Work out the finished part from the listing and answer in its coordinate system (mm). Face numbers are marked on the shaded views. A direction names the side the tool comes from. Round coordinates to 2 decimals unless told otherwise and drop trailing zeros. Write each loop counter-clockwise with the first axis right and the second up, starting at its lowest first coordinate (ties: lowest second). Pieces come first, ordered by that corner, then holes. Notation, with made-up numbers: (29, 16) -> (46, 16) arc R19 cw to (46, 39) -> close; hole circle Ø1 at (-36.5, 63). An arc over 180 degrees is marked (long way). One line per item, written item: value.
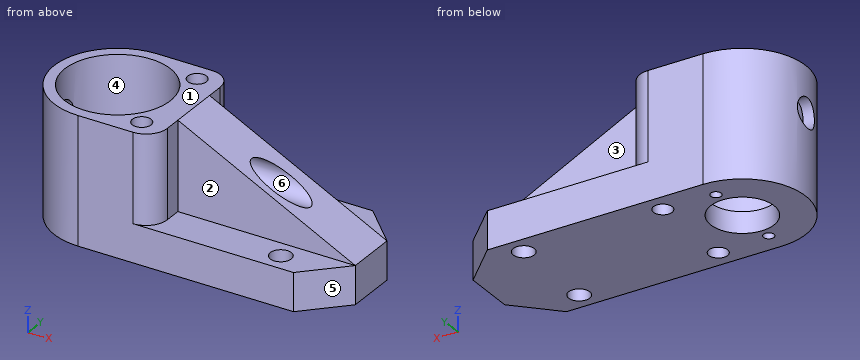
Autodesk Fusion 360 part; units mm, degrees
sketch "Sketch1" plane through (0, 0, 0) normal (0, 1, 0) x (1, 0, 0)
sketch "Sketch2" plane through (0, 0, 0) normal (0, 0, 1) x (1, 0, 0)
  line L0 (30, 15) -> (-30, 15)
  line L1 (-30, 15) -> (-30, -15)
  line L2 (-30, -15) -> (30, -15)
  line L3 (30, -15) -> (30, 15)
  line L4 (30, 15) -> (-30, -15) construction
  line L5 (-30, 15) -> (30, -15) construction
  arc A0 (-30, 15) -> (-30, -15) centre (-30, 0) ccw
  circle A1 centre (-30, 0) radius 7.5
  line L6 (21, -15) -> (30, -6)
  line L7 (21, 15) -> (30, 6)
  dimension "d1" = 60
  dimension "d2" = 30
  dimension "d3" = 15
  dimension "d4" = 9
  dimension "d5" = 9
  dimension "d6" = 9
  dimension "d7" = 9
extrude "Extrude1" add sketch "Sketch2" along normal blind 9 contours L0 L1 L2 L3 A1 L6 L7 | L1 A0 A1
sketch "Sketch3" plane through (0, 0, 9) normal (0, 0, 1) x (-1, 0, 0)
  circle A0 centre (30, 0) radius 7.5
  arc A1 (30, -15) -> (30, 15) centre (30, 0) ccw
  line L0 (30, 15) -> (-21, 15)
  line L1 (-21, 15) -> (-30, 6)
  line L2 (-30, 6) -> (-30, -6)
  line L3 (-30, -6) -> (-21, -15)
  line L4 (-21, -15) -> (30, -15)
  line L5 (12, 15) -> (12, -15)
  dimension "d10" = 18
extrude "Extrude2" add sketch "Sketch3" along normal blind 21 contours A1 L0 L4 L5
sketch "Sketch4" plane through (0, 0, 0) normal (0, 1, 0) x (1, 0, 0)
  line L0 (30, -9) -> (-12, -30)
  line L1 (-12, -30) -> (-12, -9)
  line L2 (-12, -9) -> (30, -9)
extrude "Extrude3" add sketch "Sketch4" along normal mid plane 12
sketch "Sketch5" plane through (0, 0, 30) normal (0, 0, 1) x (-1, 0, 0)
  circle A0 centre (30, 0) radius 7.5
  line L0 (12, 15) -> (12, 6)
  line L1 (12, 6) -> (12, -6)
  line L2 (12, -6) -> (12, -15)
  line L3 (12, -15) -> (30, -15)
  arc A1 (30, -15) -> (30, 15) centre (30, 0) ccw
  line L4 (30, 15) -> (12, 15)
  circle A2 centre (17.7307, -10.5) radius 2.2228
  circle A3 centre (17.7307, -10.5) radius 2.5
  dimension "d15" = 5
extrude "Extrude4" cut sketch "Sketch5" against normal blind 30 contours A2
mirror "Mirror1" about plane through (0, 0, 0) normal (0, 1, 0) of "Extrude4"
sketch "Sketch6" plane through (0, 0, 30) normal (0, 0, 1) x (-1, 0, 0)
  circle A0 centre (17.7307, 10.5) radius 2.2228
  circle A1 centre (17.7307, -10.5) radius 2.2228
  circle A2 centre (30, 0) radius 7.5
  line L0 (12, 15) -> (12, 6)
  line L1 (12, 6) -> (12, -6)
  line L2 (12, -6) -> (12, -15)
  line L3 (12, -15) -> (30, -15)
  arc A3 (30, -15) -> (30, 15) centre (30, 0) ccw
  line L4 (30, 15) -> (12, 15)
  circle A4 centre (30, 0) radius 12.5
  dimension "d20" = 25
extrude "Extrude5" cut sketch "Sketch6" against normal blind 25 contours A4
sketch "Sketch7" plane through (0, 0, 5) normal (0, 0, 1) x (-1, 0, 0)
  circle A0 centre (30, 0) radius 7.5
  circle A1 centre (30, 0) radius 12.5
  circle A2 centre (30, 10) radius 1.25
  dimension "d23" = 2.5
extrude "Extrude6" cut sketch "Sketch7" against normal blind 5 contours A2
sketch "Sketch8" plane through (0, 0, 5) normal (0, 0, 1) x (-1, 0, 0)
  circle A0 centre (30, 10) radius 1.25
  circle A1 centre (30, 0) radius 7.5
  circle A2 centre (30, 0) radius 12.5
  circle A3 centre (30, -10) radius 1.25
  dimension "d26" = 2.5
extrude "Extrude7" cut sketch "Sketch8" against normal blind 5 contours A3
sketch "Sketch9" plane through (0, 0, 0) normal (0, 0, -1) x (1, 0, 0)
  circle A0 centre (-30, -10) radius 1.25
  circle A1 centre (-30, 10) radius 1.25
  circle A2 centre (-17.7307, 10.5) radius 2.2228
  circle A3 centre (-17.7307, -10.5) radius 2.2228
  circle A4 centre (-30, 0) radius 7.5
  arc A5 (-30, 15) -> (-30, -15) centre (-30, 0) ccw
  line L0 (-30, -15) -> (21, -15)
  line L1 (21, -15) -> (30, -6)
  line L2 (30, -6) -> (30, 6)
  line L3 (30, 6) -> (21, 15)
  line L4 (21, 15) -> (-30, 15)
  circle A6 centre (15.1822, -10.5) radius 2.5
  circle A7 centre (15, 10) radius 2.5
  dimension "d29" = 5
  dimension "d30" = 5
extrude "Extrude8" cut sketch "Sketch9" against normal blind 9 contours A6
mirror "Mirror2" about plane through (0, 0, 0) normal (0, 1, 0) of "Extrude8"
sketch "Sketch10" plane through (0, 0, 0) normal (0, 0, 1) x (1, 0, 0)
fillet "Fillet1" radius 5 1 edges at (-12, 15, 19.5)
fillet "Fillet2" radius 5 1 edges at (-12, -15, 19.5)
ref_plane "WorkPlane1" through (-57, -8, 19.5) normal (1, 0, 0) x (0, 1, 0)
sketch "Sketch11" plane through (-57, -8, 19.5) normal (1, 0, 0) x (0, 1, 0)
  circle A0 centre (7.2624, -0.0862) radius 3.5
  dimension "d40" = 7
extrude "Extrude9" cut sketch "Sketch11" along normal blind 75
(1) Find section D-D on x = 22. Give the vertices of the cut face in (y, z).
Reported:
outline: (-14, 0) -> (14, 0) -> (14, 9) -> (6, 9) -> (6, 13) -> (-6, 13) -> (-6, 9) -> (-14, 9) -> close
(2) Find section A-A on z = 12. Give the vertices of the cut face in (x, y).
Reported:
outline: (-30, -15) -> (-17, -15) arc R5 ccw to (-12, -10) -> (-12, -6) -> (24, -6) -> (24, 6) -> (-12, 6) -> (-12, 10) arc R5 ccw to (-17, 15) -> (-30, 15) arc R15 ccw to start; hole circle Ø25 at (-30, 0); hole circle Ø4.45 at (-17.73, -10.5); hole circle Ø4.45 at (-17.73, 10.5)
(3) A tool of negligible diameter and unlimited length cuts with its end or side. For the marked faces 1, 2 and 3, from which of +Z, -Z, +X, -X, +Y, -Y can it reach the whole face along a straight path? Write none if from no direction.
Reported:
face 1: +Z, +X, -X, +Y, -Y
face 2: +Z, +X, -Y
face 3: +Z, +X, +Y
(4) Find section C-C on z = 2.5. Give the vertices of the cut face in (x, y), plus the area to 3 significant figures.
Reported:
outline: (-30, -15) -> (21, -15) -> (30, -6) -> (30, 6) -> (21, 15) -> (-30, 15) arc R15 ccw to start; hole circle Ø15 at (-30, 0); hole circle Ø2.5 at (-30, -10); hole circle Ø2.5 at (-30, 10); hole circle Ø4.45 at (-17.73, -10.5); hole circle Ø4.45 at (-17.73, 10.5); hole circle Ø5 at (15.18, -10.5); hole circle Ø5 at (15.18, 10.5)
area: 1,820 mm2
(5) For a pull along X with two mould halves and no side action, classify the marked faces 4, 5 and 6 as pulls with the +X half, pulls with the -X half, needs draft (parallel to the pull), parting line crosses it, or undercut.
Reported:
face 4: undercut
face 5: pulls with the +X half
face 6: needs draft
(6) Flat-ended cylindrical pins translate along their axes: pin 1 Ø4 at (x, y) = (-17.73, -10.5) entering from -Z; pin 2 Ø5 at (x, y) = (10, 7) entering from +Z; pin 3 Ø10.5 at (x, z) = (12.5, 21.5) entering from -Y; pin 4 Ø6.5 at (x, y) = (15.18, 10.5) entering from +Z. Find the tip coordinate at first contact, or state that the pin passes through.
Reported:
pin 1: passes through
pin 2: stops at z = 20.15
pin 3: stops at y = -6
pin 4: stops at z = 9
(7) Find section B-B on x = -25.5. Give the vertices of the cut face in (y, z), plus the area to 3 significant figures.
Reported:
outline: (-15, 0) -> (-6, 0) -> (-6, 5) -> (-11.66, 5) -> (-11.66, 30) -> (-15, 30) -> close; (6, 0) -> (15, 0) -> (15, 30) -> (11.66, 30) -> (11.66, 5) -> (6, 5) -> close
area: 257 mm2
(8) Consider probe 1 along Y at (x, z) = (-30, 3.55); probe 2 along X at (y, z) = (11, 15); probe 3 along X at (y, z) = (10.5, 15.75). Determine where each line is inside the solid, lowest interval first.
Reported:
probe 1: y = -15 to -11.25, -8.75 to -7.5, 7.5 to 8.75, 11.25 to 15
probe 2: x = -40.2 to -35.94, -24.06 to -19.9, -15.56 to -12.1
probe 3: x = -40.71 to -36.78, -23.22 to -19.95, -15.51 to -12.03
